from build123d import *

# Parameters (mm, degrees)
SKETCH2_R             = 2.25
BOSS_EXTRUDE1_DEPTH   = 8
M3_TAPPED_HOLE1_D     = 2.5
M3_TAPPED_HOLE1_DEPTH = 7.5
M3_TAPPED_HOLE1_TIP   = 0.751075774
M4_TAPPED_HOLE1_D     = 3.3
M4_TAPPED_HOLE1_DEPTH = 8
M4_TAPPED_HOLE1_TIP   = 0.991420021
M4_TAPPED_HOLE2_D     = 3.3
M4_TAPPED_HOLE2_DEPTH = 8
M4_TAPPED_HOLE2_TIP   = 0.991420021
FILLET1_R             = 2


with BuildPart() as part:
    # Sketch2 → Boss-Extrude1 (new body)
    with BuildSketch(Plane.XY):
        Polygon((-21.629213483, 13.033707865), (20.370786517, 13.033707865), (20.370786517, -1.966292135), (28.370786517, -1.966292135), (28.370786517, -16.966292135), (-21.629213483, -16.966292135), align=None)
        with Locations((-16.629213483, 8.033707865)):
            Circle(SKETCH2_R, mode=Mode.SUBTRACT)
        with Locations((3.370786517, 8.033707865)):
            Circle(SKETCH2_R, mode=Mode.SUBTRACT)
        with Locations((-16.629213483, -7.134831461)):
            Circle(SKETCH2_R, mode=Mode.SUBTRACT)
        with Locations((3.370786517, -7.134831461)):
            Circle(SKETCH2_R, mode=Mode.SUBTRACT)
    extrude(amount=BOSS_EXTRUDE1_DEPTH)

    # M3 Tapped Hole1
    with Locations(Plane.XY.offset(8)):
        with Locations((-2.629213483, -12.966292135), (9.370786517, -12.966292135)):
            Hole(M3_TAPPED_HOLE1_D / 2, depth=M3_TAPPED_HOLE1_DEPTH)
            with Locations((0, 0, -(M3_TAPPED_HOLE1_DEPTH + M3_TAPPED_HOLE1_TIP / 2))):  # 118° drill point
                Cone(0, M3_TAPPED_HOLE1_D / 2, M3_TAPPED_HOLE1_TIP, mode=Mode.SUBTRACT)

    # M4 Tapped Hole1
    with Locations(Plane(origin=(28.370786517, 0, 0), x_dir=(0, 0, -1), z_dir=(1, 0, 0))):
        with Locations((-4, -11.966292135)):
            Hole(M4_TAPPED_HOLE1_D / 2, depth=M4_TAPPED_HOLE1_DEPTH)
            with Locations((0, 0, -(M4_TAPPED_HOLE1_DEPTH + M4_TAPPED_HOLE1_TIP / 2))):  # 118° drill point
                Cone(0, M4_TAPPED_HOLE1_D / 2, M4_TAPPED_HOLE1_TIP, mode=Mode.SUBTRACT)

    # M4 Tapped Hole2
    with Locations(Plane.ZY.offset(21.629213483)):
        with Locations((4, -11.966292135)):
            Hole(M4_TAPPED_HOLE2_D / 2, depth=M4_TAPPED_HOLE2_DEPTH)
            with Locations((0, 0, -(M4_TAPPED_HOLE2_DEPTH + M4_TAPPED_HOLE2_TIP / 2))):  # 118° drill point
                Cone(0, M4_TAPPED_HOLE2_D / 2, M4_TAPPED_HOLE2_TIP, mode=Mode.SUBTRACT)

    # Fillet1
    fillet1_edges = [part.edges().sort_by_distance(p)[0] for p in [
        (20.370786517, -1.966292135, 4),
    ]]
    fillet(fillet1_edges, radius=FILLET1_R)


solid = part.part
Input: part model. Units: mm. Frame: model coordinates. A direction names the side the tool comes from. Round coordinates to 2 decimals unless told otherwise and drop trailing zeros. Order: outer loops, then holes, each group sorted by start corner. A loop starts at its lowest first (then second) coordinate and runs counter-clockwise, first axis right, second up.
1. Set-up query: faces 1 (the face through (-17.57, -12.97, 5.31)), 2 (the face through (-3.3, -11.91, 4.2)), 3 (the face through (20.371, 7, 4)), 4 (the face through (19.552, -11.682, 4.037)). Return all of +Z, -Z, +X, -X, +Y, -Y with unobstructed straight access to the full face (end or side cutting, diameter ignored); none if empty.
The answers:
face 1: -X
face 2: +Z
face 3: +Z, -Z, +X, +Y
face 4: +X
2. Cut plane B-B, the plane y = -8. Output: boundary loops of the cut face in (x, z).
The answers:
outline: (-21.63, 0) - (-18.71, 0) - (-18.71, 8) - (-21.63, 8) - close; (-14.55, 0) - (1.29, 0) - (1.29, 8) - (-14.55, 8) - close; (5.45, 0) - (28.37, 0) - (28.37, 8) - (5.45, 8) - close
3. Cut plane C-C, the plane z = 6.5. Output: boundary loops of the cut face in (x, y), then the cut area to 3 significant figures.
The answers:
outline: (-21.63, -16.97) - (28.37, -16.97) - (28.37, -1.97) - (22.37, -1.97) arc R2 cw to (20.37, 0.03) - (20.37, 13.03) - (-21.63, 13.03) - close; hole circle Ø4.5 at (-16.63, -7.13); hole circle Ø4.5 at (-16.63, 8.03); hole circle Ø2.5 at (-2.63, -12.97); hole circle Ø4.5 at (3.37, -7.13); hole circle Ø4.5 at (3.37, 8.03); hole circle Ø2.5 at (9.37, -12.97)
area: 1,310 mm2
4. Pin query (flat end, axial travel): P1, Ø1, axis at y = 9, z = 1.5, coming from the +X side; P2, Ø2, axis at x = -2.63, y = -12.97, coming from the +Z side. Return the tip coordinate at first contact, or that it passes through.
The answers:
P1: stops at x = 20.37
P2: stops at z = 0.35
5. Material intervals for line 1 (X direction, y = -7.25, z = 2.25); line 2 (X direction, y = -8, z = 7.75); line 3 (Y direction, x = -18.5, z = 2.25), sorted ascending.
The answers:
line 1: x = -21.63 to -18.88, -14.38 to 1.12, 5.62 to 28.37
line 2: x = -21.63 to -18.71, -14.55 to 1.29, 5.45 to 28.37
line 3: y = -16.97 to -8.38, -5.88 to 6.78, 9.28 to 13.03
6. Cut plane A-A, the plane x = -15. Output: boundary loops of the cut face in (y, z), then the cut area to 3 significant figures.
The answers:
outline: (-16.97, 0) - (-8.69, 0) - (-8.69, 8) - (-16.97, 8) - close; (-5.58, 0) - (6.48, 0) - (6.48, 8) - (-5.58, 8) - close; (9.59, 0) - (13.03, 0) - (13.03, 8) - (9.59, 8) - close; hole circle Ø3.3 at (-11.97, 4)
area: 182 mm2
7. Mould query, pull axis Y, two halves, no side actions, for faces 5 (the face through (4, -2, 8)), 6 (the face through (-18.877, 8.133, 3.944)), 7 (the face through (-1, 13.034, 4)). Classes: released by +Y, released by -Y, zero draft, split by the parting line, or undercut.
The answers:
face 5: zero draft
face 6: undercut
face 7: released by +Y
